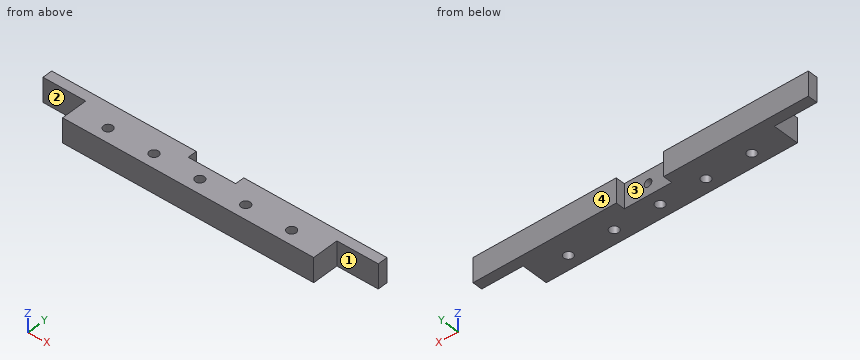
```python
from build123d import *

# Parameters (mm, degrees)
CROQUIS1_R              = 6
SALIENTE_EXTRUIR1_DEPTH = 32
CROQUIS2_R              = 5
CORTAR_EXTRUIR1_DEPTH   = 10


with BuildPart() as part:
    # Croquis1 → Saliente-Extruir1 (new body)
    with BuildSketch(Plane.XY):
        Polygon((-197.653640257, 0), (-8.534796574, 0), (-8.534796574, -12), (53.465203426, -12), (53.465203426, 0), (240.846359743, 0), (240.846359743, -13), (186.715203426, -13), (186.715203426, -47.5), (-141.784796574, -47.5), (-141.784796574, -13), (-197.653640257, -13), align=None)
        with Locations((22.465203426, -30)):
            Circle(CROQUIS1_R, mode=Mode.SUBTRACT)
        with Locations((82.465203426, -30)):
            Circle(CROQUIS1_R, mode=Mode.SUBTRACT)
        with Locations((142.465203426, -30)):
            Circle(CROQUIS1_R, mode=Mode.SUBTRACT)
        with Locations((-37.534796574, -30)):
            Circle(CROQUIS1_R, mode=Mode.SUBTRACT)
        with Locations((-97.534796574, -30)):
            Circle(CROQUIS1_R, mode=Mode.SUBTRACT)
    extrude(amount=SALIENTE_EXTRUIR1_DEPTH)

    # Croquis2 → Cortar-Extruir1 (cut)
    with BuildSketch(Plane(origin=(0, -12, 0), x_dir=(1, 0, 0), z_dir=(0, 1, 0))):
        with Locations((22.465203426, -16)):
            Circle(CROQUIS2_R)
    extrude(amount=-CORTAR_EXTRUIR1_DEPTH, mode=Mode.SUBTRACT)


solid = part.part
```
CAD build for the part. Positions are in the model's coordinates, mm. Face numbers are marked on the shaded views. A direction names the side the tool comes from. Coordinates: 2 decimals unless noted, no trailing zeros. Order: outer loops, then holes, each group sorted by start corner. A loop starts at its lowest first (then second) coordinate and runs counter-clockwise, first axis right, second up.
(1) Which spindle directions (+Z, -Z, +X, -X, +Y, -Y) get a long thin tool onto all of the face, cutting with end or side? Do the marked faces 1, 2, 3 and 4. Say none if no direction does.
Solution:
face 1: +Z, -Z, +X, -Y
face 2: +Z, -Z, -X, -Y
face 3: +Z, -Z, +Y
face 4: +Z, -Z, +X, -X, +Y
(2) Drill centre lines: L1, parallel to X at y = -27, z = 30; L2, parallel to X at y = -35, z = 30; L3, parallel to X at y = -18.5, z = 16. Where is each one in solid material? Low to high.
Solution:
L1: x = -141.78 to -102.73, -92.34 to -42.73, -32.34 to 17.27, 27.66 to 77.27, 87.66 to 137.27, 147.66 to 186.72
L2: x = -141.78 to -100.85, -94.22 to -40.85, -34.22 to 19.15, 25.78 to 79.15, 85.78 to 139.15, 145.78 to 186.72
L3: x = -141.78 to 17.47, 27.47 to 186.72
(3) Saw through at C-C, the plane x = 23. Write the cut outline in (y, z).
Solution:
outline: (-47.5, 0) - (-35.98, 0) - (-35.98, 32) - (-47.5, 32) - close; (-24.02, 0) - (-12, 0) - (-12, 11.03) - (-22, 11.03) - (-22, 20.97) - (-12, 20.97) - (-12, 32) - (-24.02, 32) - close
(4) Saw through at A-A, the plane y = -30. Write the cut outline in (x, z).
Solution:
outline: (-141.78, 0) - (-103.53, 0) - (-103.53, 32) - (-141.78, 32) - close; (-91.53, 0) - (-43.53, 0) - (-43.53, 32) - (-91.53, 32) - close; (-31.53, 0) - (16.47, 0) - (16.47, 32) - (-31.53, 32) - close; (28.47, 0) - (76.47, 0) - (76.47, 32) - (28.47, 32) - close; (88.47, 0) - (136.47, 0) - (136.47, 32) - (88.47, 32) - close; (148.47, 0) - (186.72, 0) - (186.72, 32) - (148.47, 32) - close
(5) Saw through at B-B, the plane z = 16. Write the cut outline in (x, y).
Solution:
outline: (-197.65, -13) - (-141.78, -13) - (-141.78, -47.5) - (186.72, -47.5) - (186.72, -13) - (240.85, -13) - (240.85, 0) - (53.47, 0) - (53.47, -12) - (27.47, -12) - (27.47, -22) - (17.47, -22) - (17.47, -12) - (-8.53, -12) - (-8.53, 0) - (-197.65, 0) - close; hole circle Ø12 at (-97.53, -30); hole circle Ø12 at (-37.53, -30); hole circle Ø12 at (22.47, -30); hole circle Ø12 at (82.47, -30); hole circle Ø12 at (142.47, -30)
(6) Pin check, flat tips, straight feed: pin 1 Ø15.5 at (x, y) = (-97.53, -30) entering from -Z; pin 2 Ø9.5 at (y, z) = (-36, 9) entering from -X; pin 3 Ø5 at (x, z) = (20, 17.5) entering from +Y; pin 4 Ø7 at (x, y) = (142.47, -30) entering from +Z. Stop position of each tip, or through.
Solution:
pin 1: stops at z = 0
pin 2: stops at x = -141.78
pin 3: stops at y = -12
pin 4: passes through
